Autodesk Inventor part; units mm, degrees
ref_plane "YZ Plane" through (0, 0, 0) normal (1, 0, 0) x (0, 1, 0)
ref_plane "XZ Plane" through (0, 0, 0) normal (0, 1, 0) x (-1, 0, 0)
ref_plane "XY Plane" through (0, 0, 0) normal (0, 0, 1) x (1, 0, 0)
sketch "Sketch1" plane through (0, 0, 0) normal (0, 1, 0) x (-1, 0, 0)
  line L0 (23.4545, 19) -> (23.4545, 22)
  line L1 (18.9091, 22) -> (18.9091, 19)
  line L2 (14.3636, 19) -> (14.3636, 22)
  line L3 (9.8182, 22) -> (9.8182, 19)
  line L4 (5.2727, 19) -> (5.2727, 22)
  line L5 (0.7273, 22) -> (0.7273, 19)
  line L6 (-3.8182, 19) -> (-3.8182, 22)
  line L7 (-8.3636, 22) -> (-8.3636, 19)
  line L8 (-12.9091, 19) -> (-12.9091, 22)
  line L9 (-17.4545, 22) -> (-17.4545, 19)
  line L10 (-22, 15) -> (-19, 15)
  line L11 (-19, 3) -> (-22, 3)
  line L12 (-19, -9) -> (-22, -9)
  line L13 (-22, -21) -> (-19, -21)
  line L14 (-17.4545, -25) -> (-17.4545, -28)
  line L15 (-12.9091, -28) -> (-12.9091, -25)
  line L16 (-8.3636, -25) -> (-8.3636, -28)
  line L17 (-3.8182, -28) -> (-3.8182, -25)
  line L18 (0.7273, -28) -> (0.7273, -25)
  line L19 (5.2727, -25) -> (5.2727, -28)
  line L20 (23.4545, -28) -> (23.4545, -25)
  line L21 (18.9091, -25) -> (18.9091, -28)
  line L22 (14.3636, -28) -> (14.3636, -25)
  line L23 (9.8182, -25) -> (9.8182, -28)
  line L24 (28, -21) -> (25, -21)
  line L25 (25, 15) -> (28, 15)
  line L26 (28, 3) -> (25, 3)
  line L27 (18.9091, -28) -> (23.4545, -28)
  line L28 (9.8182, -28) -> (14.3636, -28)
  line L29 (0.7273, -28) -> (5.2727, -28)
  line L30 (28, -21) -> (28, -17)
  line L31 (28, 3) -> (28, 7)
  line L32 (28, 11) -> (28, 15)
  line L33 (23.4545, 22) -> (18.9091, 22)
  line L34 (14.3636, 22) -> (9.8182, 22)
  line L35 (5.2727, 22) -> (0.7273, 22)
  line L36 (-3.8182, 22) -> (-8.3636, 22)
  line L37 (-12.9091, 22) -> (-17.4545, 22)
  line L38 (-19, 15) -> (-19, 11)
  line L39 (-19, 7) -> (-19, 3)
  line L40 (-22, 3) -> (-22, -1)
  line L41 (-22, 19) -> (-22, 15)
  line L42 (-17.4545, -28) -> (-12.9091, -28)
  line L43 (-8.3636, -28) -> (-3.8182, -28)
  line L44 (-19, -9) -> (-19, -13)
  line L45 (-19, -17) -> (-19, -21)
  line L46 (-22, -5) -> (-22, -9)
  line L47 (-22, -21) -> (-22, -25)
  line L48 (-22, -25) -> (-17.4545, -25)
  line L49 (-12.9091, -25) -> (-8.3636, -25)
  line L50 (-3.8182, -25) -> (0.7273, -25)
  line L51 (5.2727, -25) -> (9.8182, -25)
  line L52 (14.3636, -25) -> (18.9091, -25)
  line L53 (23.4545, -25) -> (25, -25)
  line L54 (25, -25) -> (25, -21)
  line L55 (25, -1) -> (25, 3)
  line L56 (25, 15) -> (25, 19)
  line L57 (25, 19) -> (23.4545, 19)
  line L58 (18.9091, 19) -> (14.3636, 19)
  line L59 (9.8182, 19) -> (5.2727, 19)
  line L60 (0.7273, 19) -> (-3.8182, 19)
  line L61 (-8.3636, 19) -> (-12.9091, 19)
  line L62 (-17.4545, 19) -> (-22, 19)
  line L63 (28, -13) -> (28, -9)
  line L64 (28, -9) -> (25, -9)
  line L65 (25, -9) -> (25, -5)
  line L66 (-19, -17) -> (-19, -13)
  line L67 (-22, -5) -> (-22, -1)
  line L68 (-19, 7) -> (-19, 11)
  line L69 (28, -17) -> (28, -13)
  line L70 (25, -5) -> (25, -1)
  line L71 (28, 7) -> (28, 11)
  point P0 (0, 0)
  point P1 (-219, 16.6364)
  point P2 (-222, -22.6364)
  point P3 (228, -22.6364)
  point P4 (-11.5, 9)
  point P5 (-11.5, 6.8182)
  point P6 (-14.5, 0.2727)
  point P7 (-11.5, -6.2727)
  point P8 (20.5, -12.8182)
  point P9 (20.5, -10.6364)
  point P10 (17.5, -3.0455)
  point P11 (17.5, -2.9545)
  point P12 (-11.5, 6.8182)
  point P13 (-14.5, 6.8182)
  point P14 (-14.5, 5)
  point P15 (-14.5, 9)
  dimension "d1" = 47
  dimension "d3" = 44
  dimension "d5" = 25
  dimension "d6" = 25
  dimension "d9" = 3
  dimension "d15" = 3
  dimension "d16" = 3
  dimension "d17" = 3
  dimension "d18" = 12
  dimension "d19" = 12
  dimension "d20" = 12
  dimension "d21" = 4
  dimension "d23" = 4.5454
extrude "Extrusion1" add sketch "Sketch1" along normal blind 3
equation "\"d1\" = wt - tt"
equation "\"d3\" = -2 * tt + ht"
equation "\"d9\" = tt"
equation "\"d15\" = tt"
equation "\"d16\" = tt"
equation "\"d17\" = tt"
equation "\"d18\" = 0.272727 * ht - 0.545455 * tt"
equation "\"d19\" = d18"
equation "\"d20\" = d18"
equation "\"d21\" = -0.181818 * tt + 0.0909091 * ht"
equation "\"d23\" = 0.0909091 * wt"
equation "\"d13\" = tt"
equation "\"wt\" = 50"
equation "\"tt\" = 3"
equation "\"tol\" = 0"
equation "\"tiroir\" = 25.4"
equation "\"nHoles\" = 101.6"
equation "\"shelfH\" = 35"
equation "\"d0\" = 0.5 * wt"
equation "\"d2\" = 0.5 * lt"
equation "\"d4\" = tt"
properties part number "base"
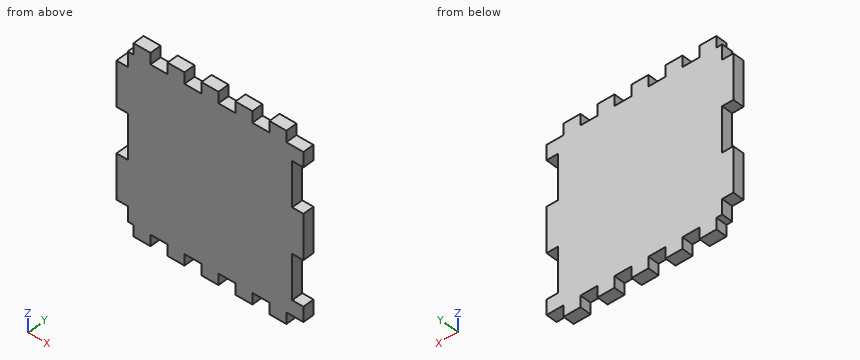
Input: part model. Units: mm. Frame: model coordinates. Give positions to 0.01 mm unless a question says otherwise; leave off trailing zeros. Order: outer loops, then holes, each group sorted by start corner. A loop starts at its lowest first (then second) coordinate and runs counter-clockwise, first axis right, second up.
1. Cut plane A-A (z = -23). Return loops of the section in (x, y).
Computed:
outline: (-25, 0) - (22, 0) - (22, 3) - (-25, 3) - close
2. Cut plane B-B (x = -7.5). Return loops of the section in (y, z).
Computed:
outline: (0, -25) - (3, -25) - (3, 19) - (0, 19) - close
3. Pin query (flat end, axial travel): pin 1 Ø0.9 at (x, y) = (20.5, 1) entering from -Z; pin 2 Ø1 at (y, z) = (2.5, -19.5) entering from +X; pin 3 Ø0.9 at (y, z) = (1, 20.5) entering from -X. Return the tip coordinate at first contact, or that it passes through.
Computed:
pin 1: stops at z = -25
pin 2: stops at x = 19
pin 3: stops at x = -23.45
4. Line query: probe 1 along X at (y, z) = (1.9, 20); probe 2 along Z at (x, y) = (0, 2.9); probe 3 along X at (y, z) = (0.2, -2.5). Output: solid intervals per line, ascending.
Computed:
probe 1: x = -23.45 to -18.91, -14.36 to -9.82, -5.27 to -0.73, 3.82 to 8.36, 12.91 to 17.45
probe 2: z = -25 to 19
probe 3: x = -25 to 22
